from build123d import *

# Parameters (mm, degrees)
ESKIZ_KONTUR_W        = 5.2
ESKIZ_KONTUR_H        = 9.2
ESKIZ_KONTUR_W_2      = 41.2
ESKIZ_KONTUR_H_2      = 20.2
PLASTINA_DEPTH        = 5
OTVERSTIYA_DEPTH      = 85.528105852
OTVERSTIYA_DEPTH_BACK = 85.528105852
ESKIZ_OTVERSTIYA_R    = 1.65


with BuildPart() as part:
    # Eskiz_kontur → Plastina (new body)
    with BuildSketch(Plane.XY):
        with BuildLine():
            Line((21.958964111, 51.343070401), (24.999994111, 4.01e-07))
            Line((24.999994111, 4.01e-07), (17, 4.01e-07))
            Line((17, 4.01e-07), (17, -5))
            Line((17, -5), (5, -5))
            Line((5, -5), (5, 0))
            Line((5, 0), (-7.35, 0))
            Line((-7.35, 0), (-7.35, 4.5))
            Line((-7.35, 4.5), (-6.1, 4.5))
            Line((-6.1, 4.5), (-6.1, 7.1))
            Line((-6.1, 7.1), (-7.35, 7.1))
            Line((-7.35, 7.1), (-7.35, 10))
            Line((-7.35, 10), (-10.65, 10))
            Line((-10.65, 10), (-10.65, 7.1))
            Line((-10.65, 7.1), (-11.9, 7.1))
            Line((-11.9, 7.1), (-11.9, 4.5))
            Line((-11.9, 4.5), (-10.65, 4.5))
            Line((-10.65, 4.5), (-10.65, 0))
            Line((-10.65, 0), (-23, 0))
            Line((-23, 0), (-23, -5))
            Line((-23, -5), (-35, -5))
            Line((-35, -5), (-35, 0))
            Line((-35, 0), (-42, 0))
            Line((-42, 0), (-43.99513, 57.7208))
            ThreePointArc((-43.99513, 57.7208), (-42.217170806, 63.034563621), (-37.389183787, 65.878463067))
            Line((-37.389183787, 65.878463067), (-3.820263787, 71.665773067))
            ThreePointArc((-3.820263787, 71.665773067), (13.620063981, 67.276975245), (21.958964111, 51.343070401))
        make_face()
        with Locations((-35.5, 16.5)):
            Rectangle(ESKIZ_KONTUR_W, ESKIZ_KONTUR_H, mode=Mode.SUBTRACT)
        with Locations((-10.15, 50)):
            Rectangle(ESKIZ_KONTUR_W_2, ESKIZ_KONTUR_H_2, mode=Mode.SUBTRACT)
    extrude(amount=PLASTINA_DEPTH)

    # Eskiz_otverstiya → Otverstiya (cut, two sides: drawn at the far end of the back side and taken through both)
    with BuildSketch(Plane.XY.offset(-OTVERSTIYA_DEPTH_BACK)):
        with Locations((-35.5, 7.5)):
            Circle(ESKIZ_OTVERSTIYA_R)
        with Locations((-34.9, 45)):
            Circle(ESKIZ_OTVERSTIYA_R)
        with Locations((-34.9, 55)):
            Circle(ESKIZ_OTVERSTIYA_R)
        with Locations((14.6, 45)):
            Circle(ESKIZ_OTVERSTIYA_R)
        with Locations((14.6, 55)):
            Circle(ESKIZ_OTVERSTIYA_R)
    extrude(amount=OTVERSTIYA_DEPTH + OTVERSTIYA_DEPTH_BACK, mode=Mode.SUBTRACT)


solid = part.part
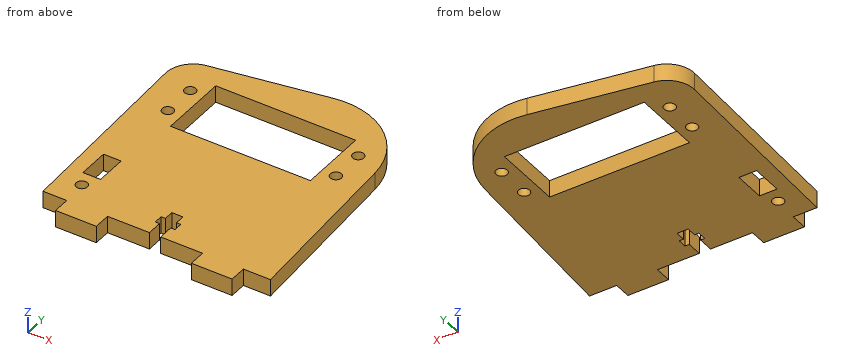
Geometry: final body of the model. Coordinates: model frame, mm. Coordinates: 2 decimals unless noted, no trailing zeros. Write each loop counter-clockwise with the first axis right and the second up, starting at its lowest first coordinate (ties: lowest second). Pieces come first, ordered by that corner, then holes. Notation, with made-up numbers: (85.25, 21.5) - (134.25, 21.5) arc R20 ccw to (134.25, 41.5) - close; hole circle Ø4 at (40.25, 28.5). An arc over 180 degrees is marked (long way). Return JSON: item names as keys, results as strings.
Item 1: Section query A-A (x = -22). Output: boundary loops of the cut face in (y, z), and give its area (3 significant figures).
Completed:
{"outline": "(0, 0) - (39.9, 0) - (39.9, 5) - (0, 5) - close; (60.1, 0) - (68.53, 0) - (68.53, 5) - (60.1, 5) - close", "area": "242 mm2"}
Item 2: Pin query (flat end, axial travel): pin 1 Ø4 at (x, y) = (-34.9, 55) entering from +Z; pin 2 Ø3 at (y, z) = (29, 1) entering from +X; pin 3 Ø2.5 at (x, z) = (19, 1.5) entering from -Y; pin 4 Ø0.8 at (y, z) = (5.5, 2) entering from -X. Return the tip coordinate at first contact, or that it passes through.
Completed:
{"pin 1": "stops at z = 5", "pin 2": "stops at x = 23.37", "pin 3": "stops at y = 0", "pin 4": "stops at x = -42.2"}
Item 3: Section query C-C (y = 13). Output: boundary loops of the cut face in (x, z).
Completed:
{"outline": "(-42.45, 0) - (-38.1, 0) - (-38.1, 5) - (-42.45, 5) - close; (-32.9, 0) - (24.23, 0) - (24.23, 5) - (-32.9, 5) - close"}
Item 4: Section query B-B (y = 45). Output: boundary loops of the cut face in (x, z), and give its area (3 significant figures).
Completed:
{"outline": "(-43.56, 0) - (-36.55, 0) - (-36.55, 5) - (-43.56, 5) - close; (-33.25, 0) - (-30.75, 0) - (-30.75, 5) - (-33.25, 5) - close; (10.45, 0) - (12.95, 0) - (12.95, 5) - (10.45, 5) - close; (16.25, 0) - (22.33, 0) - (22.33, 5) - (16.25, 5) - close", "area": "90.5 mm2"}
Item 5: Line query: L1, parallel to Y at x = 14.6, z = 3.1; L2, parallel to Y at x = -34.9, z = 1.35; L3, parallel to X at y = 53.5, z = 0.85. Output: solid intervals per line, ascending.
Completed:
{"L1": "y = -5 to 43.35, 46.65 to 53.35, 56.65 to 66.46", "L2": "y = -5 to 5.96, 9.04 to 11.9, 21.1 to 43.35, 46.65 to 53.35, 56.65 to 66.31", "L3": "x = -43.85 to -35.59, -34.21 to -30.75, 10.45 to 13.91, 15.29 to 21.72"}
Item 6: Section query D-D (x = 14.6). Output: boundary loops of the cut face in (y, z), and give its area (3 significant figures).
Completed:
{"outline": "(-5, 0) - (43.35, 0) - (43.35, 5) - (-5, 5) - close; (46.65, 0) - (53.35, 0) - (53.35, 5) - (46.65, 5) - close; (56.65, 0) - (66.46, 0) - (66.46, 5) - (56.65, 5) - close", "area": "324 mm2"}
